from build123d import *

# Parameters (mm, degrees)
SKETCH1_R           = 2.5
SKETCH1_R_2         = 8.5
BOSS_EXTRUDE1_DEPTH = 10


with BuildPart() as part:
    # Sketch1 → Boss-Extrude1 (new body)
    with BuildSketch(Plane.XY):
        with BuildLine():
            Line((-13, 20), (-40, 20))
            ThreePointArc((-40, 20), (-47.071067812, 17.071067812), (-50, 10))
            Line((-50, 10), (-50, -10))
            ThreePointArc((-50, -10), (-47.071067812, -17.071067812), (-40, -20))
            Line((-40, -20), (-13, -20))
            Line((-13, -20), (-13, -63.686733312))
            ThreePointArc((-13, -63.686733312), (0, -65), (13, -63.686733312))
            Line((13, -63.686733312), (13, -20))
            Line((13, -20), (40, -20))
            ThreePointArc((40, -20), (47.071067812, -17.071067812), (50, -10))
            Line((50, -10), (50, 10))
            ThreePointArc((50, 10), (47.071067812, 17.071067812), (40, 20))
            Line((40, 20), (13, 20))
            Line((13, 20), (13, 63.686733312))
            ThreePointArc((13, 63.686733312), (0, 65), (-13, 63.686733312))
            Line((-13, 63.686733312), (-13, 20))
        make_face()
        with Locations((-37.5, 0)):
            Circle(SKETCH1_R, mode=Mode.SUBTRACT)
        with Locations((0, -50)):
            Circle(SKETCH1_R, mode=Mode.SUBTRACT)
        with Locations((37.5, 0)):
            Circle(SKETCH1_R, mode=Mode.SUBTRACT)
        with Locations((0, 50)):
            Circle(SKETCH1_R, mode=Mode.SUBTRACT)
        Circle(SKETCH1_R_2, mode=Mode.SUBTRACT)
    extrude(amount=BOSS_EXTRUDE1_DEPTH)


solid = part.part
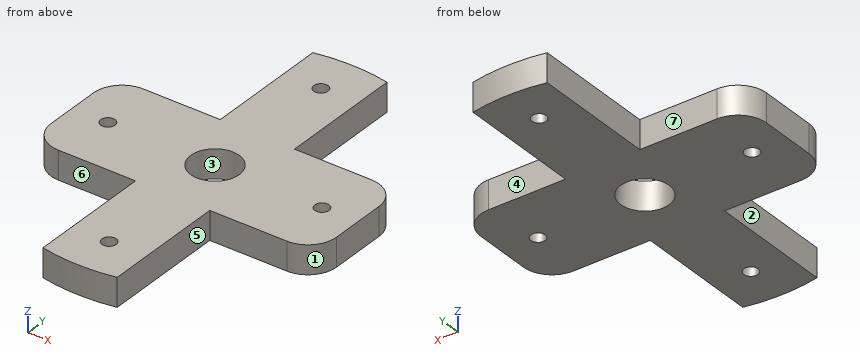
Source: CAD feature listing. Evaluate the final solid. Frame: model axes, mm. Face numbers are marked on the shaded views. A direction names the side the tool comes from. Give positions to 0.01 mm unless a question says otherwise; leave off trailing zeros. Order: outer loops, then holes, each group sorted by start corner. A loop starts at its lowest first (then second) coordinate and runs counter-clockwise, first axis right, second up. Notation, with made-up numbers: (-31, -1) -> (25, -1) arc R25 cw to (25, 19) -> close; hole circle Ø10 at (45.25, 84). An arc over 180 degrees is marked (long way). Write item = value, one per line.
Item 1: Section query B-B (y = -50). Output: boundary loops of the cut face in (x, z), then the cut area to 3 significant figures.
Check result:
outline = (-13, 0) -> (-2.5, 0) -> (-2.5, 10) -> (-13, 10) -> close; (2.5, 0) -> (13, 0) -> (13, 10) -> (2.5, 10) -> close
area = 210 mm²
Item 2: Set-up query: the marked faces 4, 5, 6 and 7. Return all of +Z, -Z, +X, -X, +Y, -Y with unobstructed straight access to the full face (end or side cutting, diameter ignored); none if empty.
Check result:
face_4 = +Z, -Z, +X, +Y
face_5 = +Z, -Z, +X, -Y
face_6 = +Z, -Z, -X, -Y
face_7 = +Z, -Z, -X, +Y
Item 3: Section query D-D (y = 0). Output: boundary loops of the cut face in (x, z).
Check result:
outline = (-50, 0) -> (-40, 0) -> (-40, 10) -> (-50, 10) -> close; (-35, 0) -> (-8.5, 0) -> (-8.5, 10) -> (-35, 10) -> close; (8.5, 0) -> (35, 0) -> (35, 10) -> (8.5, 10) -> close; (40, 0) -> (50, 0) -> (50, 10) -> (40, 10) -> close
Item 4: Section query C-C (z = 5). Output: boundary loops of the cut face in (x, y), then the cut area to 3 significant figures.
Check result:
outline = (-50, -10) arc R10 ccw to (-40, -20) -> (-13, -20) -> (-13, -63.69) arc R65 ccw to (13, -63.69) -> (13, -20) -> (40, -20) arc R10 ccw to (50, -10) -> (50, 10) arc R10 ccw to (40, 20) -> (13, 20) -> (13, 63.69) arc R65 ccw to (-13, 63.69) -> (-13, 20) -> (-40, 20) arc R10 ccw to (-50, 10) -> close; hole circle Ø5 at (-37.5, 0); hole circle Ø17 at (0, 0); hole circle Ø5 at (0, -50); hole circle Ø5 at (0, 50); hole circle Ø5 at (37.5, 0)
area = 5,930 mm²
Item 5: Ray query, probe 1 along Y at (x, z) = (0, 6.75); probe 2 along Y at (x, z) = (37.5, 2.75); probe 3 along X at (y, z) = (-28, 3.75). Return the intervals inside material, ascending.
Check result:
probe_1 = -65 to -52.5, -47.5 to -8.5, 8.5 to 47.5, 52.5 to 65
probe_2 = -20 to -2.5, 2.5 to 20
probe_3 = -13 to 13
Item 6: Section query A-A (x = 37.5). Output: boundary loops of the cut face in (y, z), then the cut area to 3 significant figures.
Check result:
outline = (-20, 0) -> (-2.5, 0) -> (-2.5, 10) -> (-20, 10) -> close; (2.5, 0) -> (20, 0) -> (20, 10) -> (2.5, 10) -> close
area = 350 mm²
Item 7: Mould query, pull axis Y, two halves, no side actions, for the marked faces 1, 2 and 3. Classes: +Y half, -Y half, draft (parallel to the pull), parting line (faces both ways), or undercut.
Check result:
face_1 = -Y half
face_2 = draft
face_3 = undercut
Item 8: Contact query for flat-ended pins moving along their axis: pin 1 (3 mm diameter, centred on y = -42, z = 7.5, fed in from +X); pin 2 (5 mm diameter, centred on x = -20, z = 4.5, fed in from -Y); pin 3 (6 mm diameter, centred on x = -30.5, z = 1.5, fed in from +Y). Output: stop coordinate, or through.
Check result:
pin_1 = 13
pin_2 = -20
pin_3 = 20
